```python
from build123d import *

# Parameters (mm, degrees)
SKETCH1_R           = 20
BOSS_EXTRUDE1_DEPTH = 32
SKETCH2_R           = 8
BOSS_EXTRUDE3_DEPTH = 20
BOSS_EXTRUDE4_START = -4
SKETCH11_R          = 8
BOSS_EXTRUDE4_DEPTH = 18


with BuildPart() as part:
    # Sketch1 → Boss-Extrude1 (new body)
    with BuildSketch(Plane(origin=(0, 0, 0), x_dir=(1, 0, 0), z_dir=(0, 1, 0))):
        with BuildLine():
            Line((-38, -36), (38, -36))
            Line((38, -36), (38, 0))
            ThreePointArc((38, 0), (0, 38), (-38, 0))
            Line((-38, 0), (-38, -36))
        make_face()
        with Locations(Location((0, 0, 0), (0, 0, 270))):
            Circle(SKETCH1_R, mode=Mode.SUBTRACT)
    extrude(amount=BOSS_EXTRUDE1_DEPTH)

    # Sketch2 → Boss-Extrude3 (add)
    with BuildSketch(Plane(origin=(0, 32, 0), x_dir=(1, 0, 0), z_dir=(0, 1, 0))):
        with BuildLine():
            Line((-16.20578503, -84), (-38.20578503, -84))
            Line((-38.20578503, -84), (-70.20578503, -84))
            Line((-70.20578503, -84), (-70.20578503, -28))
            ThreePointArc((-70.20578503, -28), (-47.848139938, -22.366161341), (-38, -1.518653771))
            Line((-38, -1.518653771), (-38, -36))
            Line((-38, -36), (-16.20578503, -36))
            Line((-16.20578503, -36), (-16.20578503, -84))
        make_face()
        with Locations(Location((-54, -42, 0), (0, 0, 270))):
            Circle(SKETCH2_R, mode=Mode.SUBTRACT)
        with Locations(Location((-54, -70, 0), (0, 0, 270))):
            Circle(SKETCH2_R, mode=Mode.SUBTRACT)
    boss_extrude3 = extrude(amount=-BOSS_EXTRUDE3_DEPTH)

    # Mirror1: Boss-Extrude3 across plane
    add(boss_extrude3.mirror(Plane(origin=(0, 0, 0), x_dir=(0, 0, 1), z_dir=(1, 0, 0))))

    # Sketch11 → Boss-Extrude4 (add)
    with BuildSketch(Plane.ZY.offset(-16.20578503).offset(BOSS_EXTRUDE4_START)):
        with BuildLine():
            Line((36, 12), (84, 12))
            Line((84, 12), (84, -48))
            ThreePointArc((84, -48), (70.446111196, -63.811911333), (52.747932498, -52.834711668))
            Line((52.747932498, -52.834711668), (36, 0))
            Line((36, 0), (36, 12))
        make_face()
        with Locations((68, -48)):
            Circle(SKETCH11_R, mode=Mode.SUBTRACT)
    boss_extrude4 = extrude(amount=-BOSS_EXTRUDE4_DEPTH)

    # Mirror2: Boss-Extrude4 across plane
    add(boss_extrude4.mirror(Plane(origin=(0, 0, 0), x_dir=(0, 0, 1), z_dir=(1, 0, 0))))


solid = part.part
```
Model file for the job. Use its own axes, mm. A direction names the side the tool comes from. Coordinates: 2 decimals unless noted, no trailing zeros. Order: outer loops, then holes, each group sorted by start corner. A loop starts at its lowest first (then second) coordinate and runs counter-clockwise, first axis right, second up. Notation, with made-up numbers: (-3.75, 62) -> (47.25, 62) arc R15 cw to (47.25, 80) -> close; hole circle Ø1 at (89.25, -29). An arc over 180 degrees is marked (long way). Answer as a JSON object with one key per item and string values. Group by question number.
1) Flat gauge pins, fed straight in: pin 1 (14.5 mm diameter, centred on y = -48, z = 68, fed in from -X); pin 2 (14.5 mm diameter, centred on y = -11.5, z = 53, fed in from +X); pin 3 (10 mm diameter, centred on x = 36.5, y = -49, fed in from -Z); pin 4 (14.5 mm diameter, centred on y = -28, z = 69.5, fed in from -X). Where does each tip first touch, or does it go through?
2) Pull direction X, two halves, no side cores. Call faces 1 (the face through (70.206, 22, 56)), 2 (the face through (20.206, -17, 60)), 3 (the face through (29.1, -42.6, 62.1)), 4 (the face through (-70.206, 22, 56)): +X half, -X half, draft (parallel to the pull), parting line (faces both ways), or undercut.
3) Cut at D-D, the plane y = -45.5. Write the cut outline in (x, z).
4) Cut at C-C, the plane z = 42. Write the cut outline in (x, y).
5) Drill centre lines: L1, parallel to X at y = 19.5, z = 42; L2, parallel to X at y = 9, z = 56.5; L3, parallel to Y at x = 26.75, z = 68. Where is each one in solid material? Low to high.
6) Which spindle directions (+Z, -Z, +X, -X, +Y, -Y) get a long thin tool onto all of the face, cutting with end or side? Do faces 5 (the face through (-38, 6, 17)), 6 (the face through (-16.206, 22, 60)), 7 (the face through (-20.206, -17, 60)). Say none if no direction does.
7) Cut at B-B, the plane y = -22. Write the cut outline in (x, z).
8) Cut at A-A, the plane x = 0. Write the cut outline in (y, z).
Check values:
{
 "1": {"pin 1": "passes through", "pin 2": "stops at x = 38.21", "pin 3": "stops at z = 49.95", "pin 4": "stops at x = -38.21"},
 "2": {"face 1": "+X half", "face 2": "undercut", "face 3": "draft", "face 4": "-X half"},
 "3": {"outline": "(-38.21, 50.42) -> (-20.21, 50.42) -> (-20.21, 60.4) -> (-38.21, 60.4) -> close; (-38.21, 75.6) -> (-20.21, 75.6) -> (-20.21, 84) -> (-38.21, 84) -> close; (20.21, 50.42) -> (38.21, 50.42) -> (38.21, 60.4) -> (20.21, 60.4) -> close; (20.21, 75.6) -> (38.21, 75.6) -> (38.21, 84) -> (20.21, 84) -> close"},
 "4": {"outline": "(-70.21, 12) -> (-62, 12) -> (-62, 32) -> (-70.21, 32) -> close; (-46, 12) -> (-38.21, 12) -> (-38.21, -18.93) -> (-20.21, -18.93) -> (-20.21, 12) -> (-16.21, 12) -> (-16.21, 32) -> (-46, 32) -> close; (16.21, 12) -> (20.21, 12) -> (20.21, -18.93) -> (38.21, -18.93) -> (38.21, 12) -> (46, 12) -> (46, 32) -> (16.21, 32) -> close; (62, 12) -> (70.21, 12) -> (70.21, 32) -> (62, 32) -> close"},
 "5": {"L1": "x = -70.21 to -62, -46 to -16.21, 16.21 to 46, 62 to 70.21", "L2": "x = -38.21 to -20.21, 20.21 to 38.21", "L3": "y = -64 to -56, -40 to 32"},
 "6": {"face 5": "-Z, -X, -Y", "face 6": "+Z, +Y, -Y", "face 7": "+Z, -Y"},
 "7": {"outline": "(-38.21, 42.97) -> (-20.21, 42.97) -> (-20.21, 84) -> (-38.21, 84) -> close; (20.21, 42.97) -> (38.21, 42.97) -> (38.21, 84) -> (20.21, 84) -> close"},
 "8": {"outline": "(0, -38) -> (32, -38) -> (32, -20) -> (0, -20) -> close; (0, 20) -> (32, 20) -> (32, 36) -> (0, 36) -> close"}
}
